Could you check a few things on this model? Use its own coordinates, in mm. A direction names the side the tool comes from. Give positions to 0.01 mm unless a question says otherwise; leave off trailing zeros. Loops run counter-clockwise (first coordinate to the right, second up) from the corner with the lowest first, then second, coordinate; pieces in that order, holes last. Notation, with made-up numbers: M 31.5,3.5 L 38.5,3.5 A22 ccw 38.5,30.5 Z; hole C 77,29.25 d4. An arc over 180 degrees is marked long. Answer in a Markdown table with one row per item. Add a question column.
1. Thinking about a two-plate mould opening in X: for faces 1 (the flat face through (21, 2, -20)), 2 (the flat face through (4, 2, -26)), 3 (the flat face through (0, 2, -13)), which applies, released by +X, released by -X, zero draft, split by the parting line, or undercut?
2. If we section it at C-C on y = 3.4: List the corners of the cut face in (x, z) for me.
3. Which directions (+Z, -Z, +X, -X, +Y, -Y) give clear straight access to the entire face, cutting with the end or side of a thin tool? Please do faces 4 (the flat face through (7, 2, -18)), 5 (the flat face through (18, 2, -24)), 6 (the flat face through (13, 2, 0)).
4. If we section it at A-A on z = -18.75: List the corners of the cut face in (x, y) for me, then the cut area to 3 significant figures.
5. I need wall thicknesses on line 1 along X through (y, z) = (2.2, -18.25); line 2 along X through (y, z) = (2.3, -13); line 3 along Z through (x, y) = (9, 1.25). Which ranges of each line are inside material? Lowest first, please. Write a range as from..to.
6. If we section it at D-D on x = 11.75: List the corners of the cut face in (y, z) for me, then the cut area to 3 significant figures.
7. If we section it at B-B on x = 20: List the corners of the cut face in (y, z) for me.
8. I'm going to push a flat-ended pin straight in: pin 1 Ø1.5 at (x, y) = (14.5, 1.5) entering from -Z. Where does the tip first touch, or does it pass through?
```python
from build123d import *

# Parameters (mm, degrees)
EXTRUDE_1_DEPTH = 5


with BuildPart() as part:
    # 草图1 → 凸台-拉伸1 (new body)
    with BuildSketch(Plane(origin=(0, 0, 0), x_dir=(1, 0, 0), z_dir=(0, 1, 0))):
        Polygon((0, 26), (0, 0), (26, 0), (26, 26), (18, 26), (18, 21), (21, 21), (21, 18), (18, 18), (18, 8), (8, 8), (8, 18), (5, 18), (5, 21), (8, 21), (8, 26), align=None)
    extrude(amount=EXTRUDE_1_DEPTH)


solid = part.part
```
Results:
| question | item | result |
|---|---|---|
| 1 | face 1 | undercut |
| 1 | face 2 | zero draft |
| 1 | face 3 | released by -X |
| 2 | outline | M 0,-26 L 8,-26 L 8,-21 L 5,-21 L 5,-18 L 8,-18 L 8,-8 L 18,-8 L 18,-18 L 21,-18 L 21,-21 L 18,-21 L 18,-26 L 26,-26 L 26,0 L 0,0 Z |
| 3 | face 4 | +Y, -Y |
| 3 | face 5 | -Z, +Y, -Y |
| 3 | face 6 | +Z, +X, -X, +Y, -Y |
| 4 | outline | M 0,0 L 5,0 L 5,5 L 0,5 Z; M 21,0 L 26,0 L 26,5 L 21,5 Z |
| 4 | area | 50.0 mm2 |
| 5 | line 1 | 0..5, 21..26 |
| 5 | line 2 | 0..8, 18..26 |
| 5 | line 3 | -8..0 |
| 6 | outline | M 0,-8 L 5,-8 L 5,0 L 0,0 Z |
| 6 | area | 40.0 mm2 |
| 7 | outline | M 0,-26 L 5,-26 L 5,-21 L 0,-21 Z; M 0,-18 L 5,-18 L 5,0 L 0,0 Z |
| 8 | pin 1 | z = -8 |
